Check sheet for the drawn part. Datum: minimum x, y, z corner. Units: mm. Coordinates: 2 decimals unless noted, no trailing zeros. Write each loop counter-clockwise with the first axis right and the second up, starting at its lowest first coordinate (ties: lowest second). Pieces come first, ordered by that corner, then holes. Notation, with made-up numbers: (64.5, 28) -> (72.5, 28) arc R9 cw to (72.5, 33) -> close; hole circle Ø3 at (73.5, -25.5). An arc over 180 degrees is marked (long way). Answer in a Markdown table with one row per item. Add a question column.
Q1. Section check A-A, the plane y = 1.7. Record the boundary of the cut face in (x, z) (1 decimal).
Q2. Section check B-B, the plane x = 44. Record the boundary of the cut face in (y, z) (1 decimal).
Q3. Gauge pin test, flat ends, axial feed: P1, Ø1.5, axis at x = 71.5, y = 2, coming from the -Z side; P2, Ø1.5, axis at y = 2.5, z = 35.5, coming from the -X side; P3, Ø2.5, axis at y = 1, z = 43.5, coming from the +X side; P4, Ø2.5, axis at x = 95.5, y = 1.5, coming from the +Z side. Record the tip position at first contact, or that the pin passes through.
Q4. Section check C-C, the plane z = 43.5. Record the boundary of the cut face in (x, y).
Q5. Section check D-D, the plane z = 11. Record the boundary of the cut face in (x, y).
Q6. Thickness scan on line 1 (X direction, y = 1.95, z = 33); line 2 (Y direction, x = 126, z = 117); line 3 (Z direction, x = 45.5, y = 1.5) (1 decimal). Record the ranges inside material, lowest first.
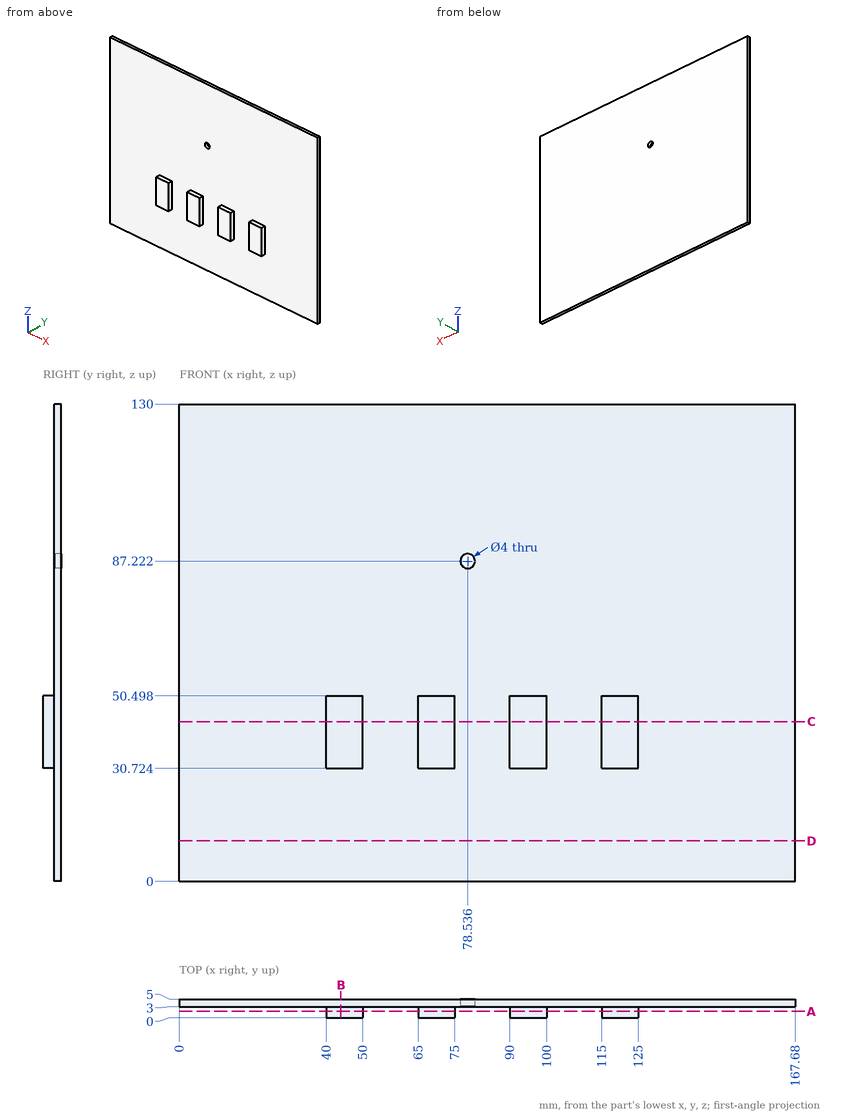
Calculated:
| question | item | result |
|---|---|---|
| 1 | outline | (40, 30.7) -> (50, 30.7) -> (50, 50.5) -> (40, 50.5) -> close; (65, 30.7) -> (75, 30.7) -> (75, 50.5) -> (65, 50.5) -> close; (90, 30.7) -> (100, 30.7) -> (100, 50.5) -> (90, 50.5) -> close; (115, 30.7) -> (125, 30.7) -> (125, 50.5) -> (115, 50.5) -> close |
| 2 | outline | (0, 30.7) -> (3, 30.7) -> (3, 0) -> (5, 0) -> (5, 130) -> (3, 130) -> (3, 50.5) -> (0, 50.5) -> close |
| 3 | P1 | stops at z = 30.72 |
| 3 | P2 | stops at x = 0 |
| 3 | P3 | stops at x = 125 |
| 3 | P4 | stops at z = 50.5 |
| 4 | outline | (0, 3) -> (40, 3) -> (40, 0) -> (50, 0) -> (50, 3) -> (65, 3) -> (65, 0) -> (75, 0) -> (75, 3) -> (90, 3) -> (90, 0) -> (100, 0) -> (100, 3) -> (115, 3) -> (115, 0) -> (125, 0) -> (125, 3) -> (167.68, 3) -> (167.68, 5) -> (0, 5) -> close |
| 5 | outline | (0, 3) -> (167.68, 3) -> (167.68, 5) -> (0, 5) -> close |
| 6 | line 1 | x = 40 to 50, 65 to 75, 90 to 100, 115 to 125 |
| 6 | line 2 | y = 3 to 5 |
| 6 | line 3 | z = 30.7 to 50.5 |
